The listing builds one solid part. Answer for the finished solid, in the listing's coordinates (mm). Round coordinates to 2 decimals unless told otherwise and drop trailing zeros. Write each loop counter-clockwise with the first axis right and the second up, starting at its lowest first coordinate (ties: lowest second). Pieces come first, ordered by that corner, then holes. Notation, with made-up numbers: (24.25, 38) - (59.25, 38) arc R24 ccw to (59.25, 48) - close; hole circle Ø9 at (50, -17.5). An arc over 180 degrees is marked (long way). Answer in a Markdown table with one row per item.
from build123d import *

# Parameters (mm, degrees)
F0_R     = 27
F1_DEPTH = 5
F2_R     = 2
F3_R     = 1.5
F4_DEPTH = 5.001


with BuildPart() as f1:
    # F0 (on Top) → F1 (new body)
    with BuildSketch(Plane.XY):
        Circle(F0_R)
    extrude(amount=F1_DEPTH)

    # F2
    f2_edges = [f1.edges().sort_by_distance(p)[0] for p in [
        (-27, 0, 5),
    ]]
    fillet(f2_edges, radius=F2_R)

    # F3 (on face) → F4 (cut, through all)
    with BuildSketch(Plane(origin=(0, 0, 0), x_dir=(1, 0, 0), z_dir=(0, 0, -1))):
        with Locations((0, 13)):
            Circle(F3_R)
        with Locations((0, -13)):
            Circle(F3_R)
    extrude(amount=-F4_DEPTH, mode=Mode.SUBTRACT)


solid = f1.part
(1) Find the intervals of material crossed by line 1 (Y direction, x = 0, z = 2.45); line 2 (X direction, y = 13, z = 2.55); line 3 (X direction, y = -12.5, z = 0.8), in increasing order.
Checked values:
| item | result |
|---|---|
| line 1 | y = -27 to -14.5, -11.5 to 11.5, 14.5 to 27 |
| line 2 | x = -23.66 to -1.5, 1.5 to 23.66 |
| line 3 | x = -23.93 to -1.41, 1.41 to 23.93 |
(2) Section A-A (x = 0) is taken. Give the vertices of the cut face in (y, z).
Checked values:
| item | result |
|---|---|
| outline | (-27, 0) - (-14.5, 0) - (-14.5, 5) - (-25, 5) arc R2 ccw to (-27, 3) - close; (-11.5, 0) - (11.5, 0) - (11.5, 5) - (-11.5, 5) - close; (14.5, 0) - (27, 0) - (27, 3) arc R2 ccw to (25, 5) - (14.5, 5) - close |
(3) Section B-B (z = 1.75) is taken. Give the vertices of the cut face in (x, y), and give its area (3 significant figures).
Checked values:
| item | result |
|---|---|
| outline | circle Ø54 at (0, 0); hole circle Ø3 at (0, -13); hole circle Ø3 at (0, 13) |
| area | 2,280 mm2 |
(4) For a pull along X with two mould halves and no side action, classify faces 1 (the cylindrical face through (-5.85, -26.36, 1.48)), 2 (the cylindrical face through (-0.325, -11.536, 2.465)), 3 (the flat face through (0, 0, 0)), 4 (the cylindrical face through (-0.325, 14.464, 2.465)) as pulls with the +X half, pulls with the -X half, needs draft (parallel to the pull), parting line crosses it, or undercut.
Checked values:
| item | result |
|---|---|
| face 1 | parting line crosses it |
| face 2 | undercut |
| face 3 | needs draft |
| face 4 | undercut |
(5) Flat-ended cylindrical pins translate along their axes: pin 1 (3 mm diameter, centred on y = 7, z = 1, fed in from +X); pin 2 (1 mm diameter, centred on y = 1, z = 1.5, fed in from +X). Find the tip coordinate at first contact, or state that the pin passes through.
Checked values:
| item | result |
|---|---|
| pin 1 | stops at x = 26.43 |
| pin 2 | stops at x = 27 |
